Input: part model. Units: mm. Frame: model coordinates. A direction names the side the tool comes from. Coordinates: 2 decimals unless noted, no trailing zeros. Write each loop counter-clockwise with the first axis right and the second up, starting at its lowest first coordinate (ties: lowest second). Pieces come first, ordered by that corner, then holes. Notation, with made-up numbers: (-6.75, 70.25) - (14.25, 70.25) arc R12 cw to (14.25, 90.25) - close; hole circle Ø1 at (-15.75, 24). An arc over 180 degrees is marked (long way). Put each result on its own line as item: value. Start each with the question number.
1. Cut plane C-C, the plane x = -16. Return loops of the section in (y, z).
2. Pin query (flat end, axial travel): pin 1 (22.5 mm diameter, centred on y = 0, z = 0, fed in from +X); pin 2 (3 mm diameter, centred on y = -8.23, z = 4.75, fed in from +X); pin 3 (4 mm diameter, centred on x = -12.5, z = -25.5, fed in from -Y); pin 4 (5 mm diameter, centred on x = -22, z = -28.5, fed in from -Y). Return the tip coordinate at first contact, or that it passes through.
3. Cut plane A-A, the plane y = 0. Return loops of the section in (x, z).
4. Line query: line 1 (Z direction, x = -2, y = 0); line 2 (Z direction, x = 2, y = 8); line 3 (X direction, y = 25, z = -30.5). Output: solid intervals per line, ascending.
5. Cut plane D-D, the plane y = 32.5. Return loops of the section in (x, z), and give its area (3 significant figures).
6. Access query for faces 4 (the cylindrical face through (-15.78, 18.28, 28.67)), 5 (the cylindrical face through (2, 0, 3)), 6 (the cylindrical face through (5.535, 11.923, 3.755)), 7 (the flat face through (3, 38.3, -8.7)). Directions: +Z, -Z, +X, -X, +Y, -Y. A direction counts if a zero-diameter tool reaches every point of the face in a straight line with its end or side. Return the directions, or none.
7. Cut plane B-B, the plane z = -4.75. Return loops of the section in (x, y).
8. Pull-direction query (Z, two-part tool) for faces 1 (the cylindrical face through (1.521, 9.579, 6.224)), 2 (the flat face through (-27, -38.3, -8.7)), 3 (the cylindrical face through (-29.54, -8.67, -39.05)); classes: released by +Z, released by -Z, zero draft, split by the parting line, or undercut.
from build123d import *

# Parameters (mm, degrees)
ESQUISSE2_W             = 5
ESQUISSE2_H             = 12.5
ESQUISSE3_R             = 2
ENL_V_MAT_EXTRU_1_DEPTH = 36
ESQUISSE4_R             = 3
ENL_V_MAT_EXTRU_2_DEPTH = 36


with BuildPart() as part:
    # Esquisse1 → Révolution1 (revolve)
    with BuildSketch(Plane.XY):
        Polygon((0, 34), (0, 0), (8, 0), (8, 40), (3, 40), (3, 39), (-27, 39), (-27, 40), (-32, 40), (-32, 34), align=None)
    revolve(axis=Axis((-49.644499027, 0, 0), (1, 0, 0)))

    # Esquisse2 → Enlèvement de matière-Révolution1 (revolve, cut)
    with BuildSketch(Plane.XY):
        with Locations((5.5, 6.25)):
            Rectangle(ESQUISSE2_W, ESQUISSE2_H)
    revolve(axis=Axis((0, 0, 0), (1, 0, 0)), mode=Mode.SUBTRACT)

    # Esquisse3 → Enlèv. mat.-Extru.1 (cut, through all)
    with BuildSketch(Plane(origin=(3, 0, 0), x_dir=(0, 0, -1), z_dir=(1, 0, 0))):
        with Locations((4.75, 8.227241336)):
            Circle(ESQUISSE3_R)
        with Locations((-4.75, 8.227241336)):
            Circle(ESQUISSE3_R)
        with Locations((4.75, -8.227241336)):
            Circle(ESQUISSE3_R)
        with Locations((-4.75, -8.227241336)):
            Circle(ESQUISSE3_R)
    extrude(amount=-ENL_V_MAT_EXTRU_1_DEPTH, mode=Mode.SUBTRACT)

    # Esquisse4 → Enlèv. mat.-Extru.2 (cut, through all)
    with BuildSketch(Plane(origin=(3, 0, 0), x_dir=(0, 0, -1), z_dir=(1, 0, 0))):
        Circle(ESQUISSE4_R)
    extrude(amount=-ENL_V_MAT_EXTRU_2_DEPTH, mode=Mode.SUBTRACT)


solid = part.part
Report:
1. outline: circle Ø78 at (0, 0); hole circle Ø68 at (0, 0)
2. pin 1: stops at x = 3
2. pin 2: passes through
2. pin 3: stops at y = -31.12
2. pin 4: stops at y = -29.07
3. outline: (-32, -40) - (-27, -40) - (-27, -39) - (3, -39) - (3, -40) - (8, -40) - (8, -12.5) - (3, -12.5) - (3, -3) - (0, -3) - (0, -34) - (-32, -34) - close; (-32, 34) - (0, 34) - (0, 3) - (3, 3) - (3, 12.5) - (8, 12.5) - (8, 40) - (3, 40) - (3, 39) - (-27, 39) - (-27, 40) - (-32, 40) - close
4. line 1: z = -39 to -34, 34 to 39
4. line 2: z = -38.17 to -6.74, -2.76 to 2.76, 6.74 to 38.17
4. line 3: x = -32 to -27, 3 to 8
5. outline: (-32, -23.32) - (-27, -23.32) - (-27, -21.56) - (3, -21.56) - (3, -23.32) - (8, -23.32) - (8, 23.32) - (3, 23.32) - (3, 21.56) - (-27, 21.56) - (-27, 23.32) - (-32, 23.32) - (-32, 9.99) - (0, 9.99) - (0, -9.99) - (-32, -9.99) - close
5. area: 1,120 mm^2
6. face 4: -X
6. face 5: +X, -X
6. face 6: +X
6. face 7: none
7. outline: (-32, -39.72) - (-27, -39.72) - (-27, -38.71) - (3, -38.71) - (3, -39.72) - (8, -39.72) - (8, -11.56) - (3, -11.56) - (3, -10.23) - (0, -10.23) - (0, -33.67) - (-32, -33.67) - close; (-32, 33.67) - (0, 33.67) - (0, 10.23) - (3, 10.23) - (3, 11.56) - (8, 11.56) - (8, 39.72) - (3, 39.72) - (3, 38.71) - (-27, 38.71) - (-27, 39.72) - (-32, 39.72) - close; (0, -6.23) - (3, -6.23) - (3, 6.23) - (0, 6.23) - close
8. face 1: undercut
8. face 2: zero draft
8. face 3: split by the parting line
